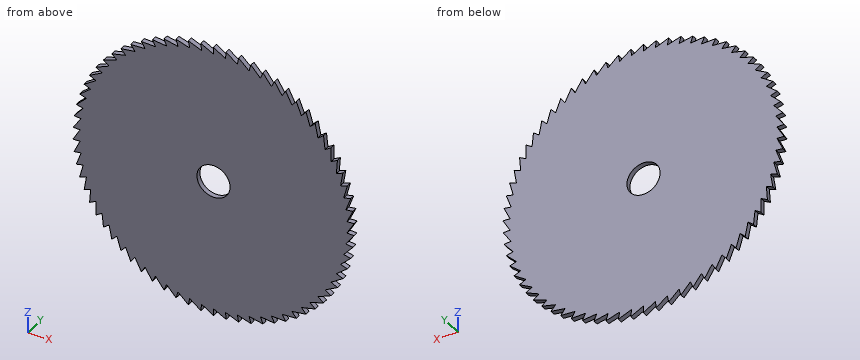
```python
from build123d import *

# Parameters (mm, degrees)
SKETCH_1_R               = 25.5
SKETCH_1_R_2             = 3
EXTRUDE_1_DEPTH          = 0.9
CUT_EXTRUDE_2_DEPTH      = 0.9
PATTERN_CIRCULAR_1_COUNT = 70


with BuildPart() as part:
    # 스케치1 → 보스-돌출1 (new body)
    with BuildSketch(Plane(origin=(0, 0, 0), x_dir=(1, 0, 0), z_dir=(0, 1, 0))):
        with Locations(Location((0, 0, 0), (0, 0, 270))):
            Circle(SKETCH_1_R)
        with Locations(Location((0, 0, 0), (0, 0, 270))):
            Circle(SKETCH_1_R_2, mode=Mode.SUBTRACT)
    extrude(amount=EXTRUDE_1_DEPTH)

    # 스케치3 → 컷-돌출2 (cut)
    with BuildSketch(Plane(origin=(0, 0.9, 0), x_dir=(1, 0, 0), z_dir=(0, 1, 0))):
        Polygon((0, 25.5), (0, 24.2), (3.797752252, 26.174934679), (0, 26.174934679), align=None)
    cut_extrude_2 = extrude(amount=-CUT_EXTRUDE_2_DEPTH, mode=Mode.SUBTRACT)

    # 원형 패턴1: 컷-돌출2 ×70 about axis
    pattern_circular_1_axis = Axis((0, 0, 0), (0, 1, 0))
    for i in range(1, PATTERN_CIRCULAR_1_COUNT):
        add(cut_extrude_2.rotate(pattern_circular_1_axis, i * 360 / PATTERN_CIRCULAR_1_COUNT), mode=Mode.SUBTRACT)


solid = part.part
```
Read the model definition and answer for the solid it produces. Units are mm, in the model's axes. Coordinates: 2 decimals unless noted, no trailing zeros. Loops run counter-clockwise (first coordinate to the right, second up) from the corner with the lowest first, then second, coordinate; pieces in that order, holes last.
(1) The part is cut by section C-C (z = 8.5). Determine the outline of the cut face in (x, y).
Solution:
outline: (-23.48, 0) - (23.19, 0) - (23.19, 0.9) - (-23.48, 0.9) - close
(2) The part is cut by section B-B (x = 7.5). Determine the outline of the cut face in (y, z), and give its area (3 significant figures).
Solution:
outline: (0, -23.55) - (0.9, -23.55) - (0.9, 23.77) - (0, 23.77) - close
area: 42.6 mm2
(3) Consider line 1 along X through (y, z) = (0.6, 0); line 2 along X through (y, z) = (0.5, -21); line 3 along Z through (x, y) = (2, 0.35). Determine where each line is inside the solid, lowest interval first.
Solution:
line 1: x = -24.8 to -3, 3 to 24.8
line 2: x = -13.51 to -12.55, -12.27 to 12.55
line 3: z = -25.24 to -2.24, 2.24 to 24.21
(4) The part is cut by section A-A (z = 0). Determine the outline of the cut face in (x, y), and give its area (3 significant figures).
Solution:
outline: (-24.8, 0) - (-3, 0) - (-3, 0.9) - (-24.8, 0.9) - close; (3, 0) - (24.8, 0) - (24.8, 0.9) - (3, 0.9) - close
area: 39.2 mm2
